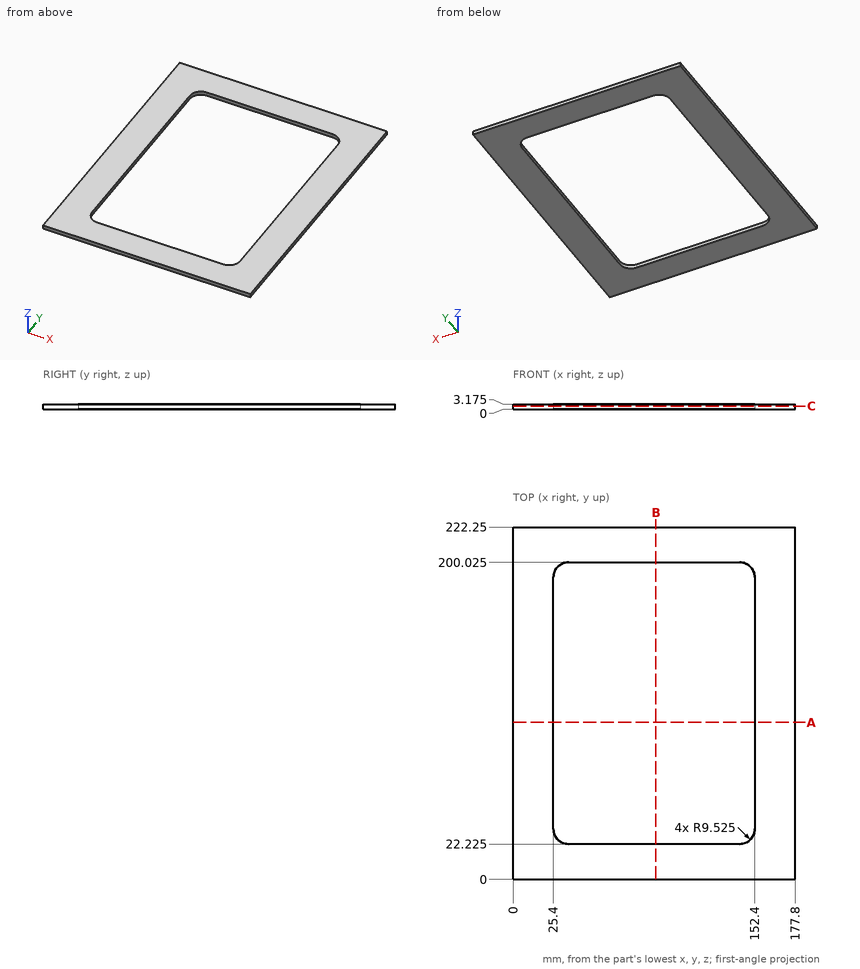
Answer from the drawing. Dimensions are ordinates in mm from the lowest x, y and z of the part. Give positions to 0.01 mm unless a question says otherwise; leave off trailing zeros. Order: outer loops, then holes, each group sorted by start corner. A loop starts at its lowest first (then second) coordinate and runs counter-clockwise, first axis right, second up. Notation, with made-up numbers: (2, 11) - (27, 11) arc R5 ccw to (27, 18) - close; hole circle Ø4 at (-36, -31.5). An arc over 180 degrees is marked (long way). One line per item, written item: value. Start each with the question number.
1. Consider line 1 (Y direction, x = 111, z = 0.35) (3 decimals); line 2 (X direction, y = 164.5, z = 1.1); line 3 (Y direction, x = 32, z = 2.35). Determine where each line is inside the solid, lowest interval first.
2. This flat-tipped pin is pushed along its axis until it touches: pin 1 Ø1.5 at (x, z) = (19.5, 3) entering from -Y. Where does it stop, or does it pass through?
3. Section C-C, the plane z = 1.8 is taken. Write down the section's boundary in (x, y) (3 decimals).
4. Section A-A, the plane y = 99 is taken. Write down the section's boundary in (x, z) (3 decimals).
5. Section B-B, the plane x = 90 is taken. Write down the section's boundary in (y, z) (3 decimals).
Filled sheet:
1. line 1: 0 to 22.225, 200.025 to 222.25
1. line 2: 0 to 25.4, 152.4 to 177.8
1. line 3: 0 to 22.69, 199.56 to 222.25
2. pin 1: y = 0
3. outline: (0, 0) - (177.8, 0) - (177.8, 222.25) - (0, 222.25) - close; hole (25.4, 31.75) arc R9.525 ccw to (34.925, 22.225) - (142.875, 22.225) arc R9.525 ccw to (152.4, 31.75) - (152.4, 190.5) arc R9.525 ccw to (142.875, 200.025) - (34.925, 200.025) arc R9.525 ccw to (25.4, 190.5) - close
4. outline: (0, 0) - (25.4, 0) - (25.4, 3.175) - (0, 3.175) - close; (152.4, 0) - (177.8, 0) - (177.8, 3.175) - (152.4, 3.175) - close
5. outline: (0, 0) - (22.225, 0) - (22.225, 3.175) - (0, 3.175) - close; (200.025, 0) - (222.25, 0) - (222.25, 3.175) - (200.025, 3.175) - close
